Job drawing, mm, ordinate dimensions from the low corner. One solid piece. Round coordinates to 2 decimals unless told otherwise and drop trailing zeros. Loops run counter-clockwise (first coordinate to the right, second up) from the corner with the lowest first, then second, coordinate; pieces in that order, holes last. Notation, with made-up numbers: M -23,22.5 L 0,22.5 A16 ccw 0,35.5 Z; hole C 57.5,37 d4. An arc over 180 degrees is marked long. Put each result on its own line as item: value. Start each with the question number.
1) Slice it at B-B on y = 25.4. Give the cut face in (x, z).
2) Slice it at A-A on z = 32. Give the cut face in (x, y), then the cut area to 3 significant figures.
3) Drop flat-ended pins along their axis: pin 1 Ø10 at (x, y) = (24.5, 22.5) entering from +Z; pin 2 Ø1.5 at (y, z) = (21, 25) entering from -X; pin 3 Ø4 at (x, z) = (24.5, 11) entering from -Y; pin 4 Ø8 at (x, z) = (36.5, 9.5) entering from +Y. Give the stop position or say it passes through.
4) Pull direction Y, two halves, no side cores. Call the marked faces 1, 2 and 3: +Y half, -Y half, draft (parallel to the pull), parting line (faces both ways), or undercut.
5) Probe line 1 along X through (y, z) = (25, 34); line 2 along Z through (x, y) = (23, 24); line 3 along X through (y, z) = (30, 30.5). List the from-to ranges inside material, lowest first.
6) Slice it at D-D on z = 8. Give the cut face in (x, y), then the cut area to 3 significant figures.
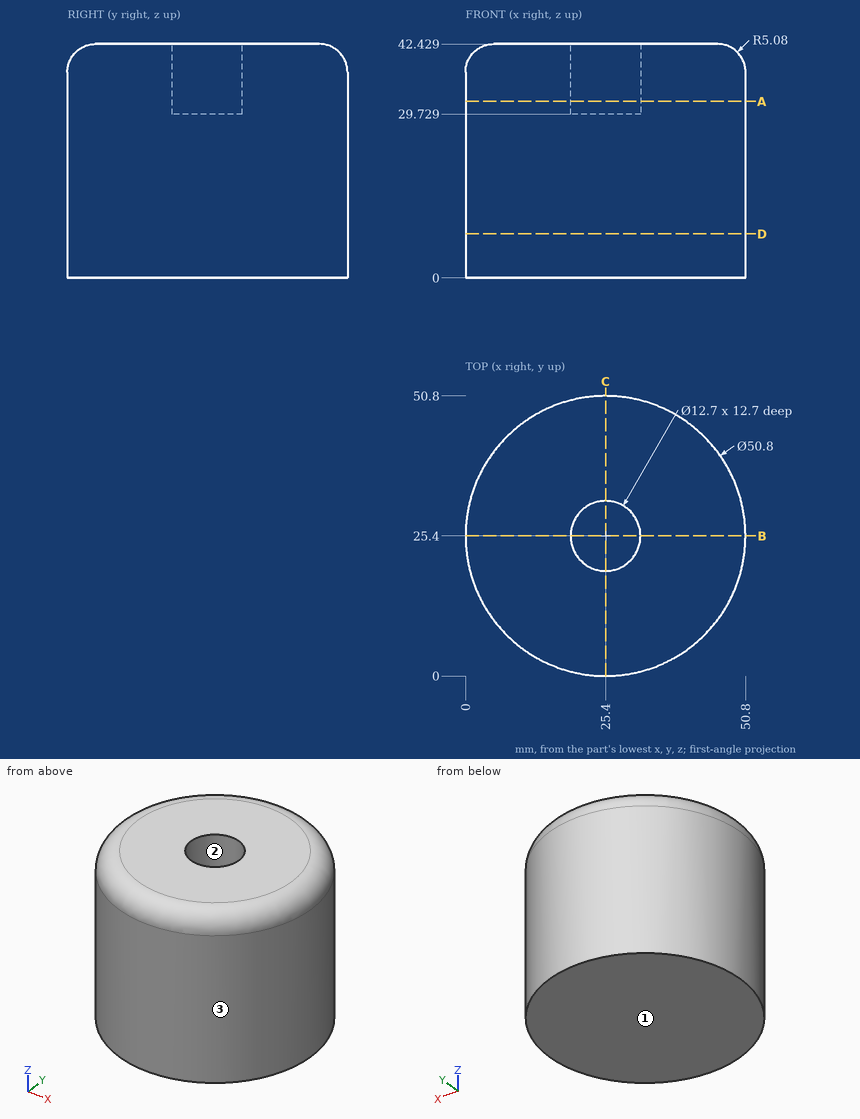
Recorded:
1. outline: M 0,0 L 50.8,0 L 50.8,37.35 A5.08 ccw 45.72,42.43 L 31.75,42.43 L 31.75,29.73 L 19.05,29.73 L 19.05,42.43 L 5.08,42.43 A5.08 ccw 0,37.35 Z
2. outline: C 25.4,25.4 d50.8; hole C 25.4,25.4 d12.7
2. area: 1,900 mm2
3. pin 1: stops at z = 42.43
3. pin 2: stops at x = 0.26
3. pin 3: stops at y = 0
3. pin 4: stops at y = 49.79
4. face 1: draft
4. face 2: undercut
4. face 3: parting line
5. line 1: x = 0 to 19.06, 31.74 to 50.8
5. line 2: z = 0 to 29.73
5. line 3: x = 0.42 to 21.02, 29.78 to 50.38
6. outline: C 25.4,25.4 d50.8
6. area: 2,030 mm2
